The listing builds one solid part. Answer for the finished solid, in the listing's coordinates (mm). Give positions to 0.01 mm unless a question says otherwise; leave off trailing zeros. Order: outer loops, then holes, each group sorted by start corner. A loop starts at its lowest first (then second) coordinate and runs counter-clockwise, first axis right, second up. Notation, with made-up numbers: (44.5, 53) - (53.5, 53) arc R23 ccw to (53.5, 70) - close; hole circle Ø5 at (30, 58.5). An arc over 180 degrees is marked (long way). Answer as CSV lines item,"result". Start each with the question number.
1. Section A-A on z = 0 is taken. Give the vertices of the cut face in (x, y) (3 decimals).
2. Determine the mould class of faces 1 (the flat face through (-8.5, -3, -19)), 2 (the cylindrical face through (-7.3, 17.5, -7.3)), 3 (the cylindrical face through (-7.81, -4.58, 20.65)) for opening direction Y: +Y half, -Y half, draft (parallel to the pull), parting line (faces both ways), or undercut.
3. Flat-ended cylindrical pins translate along their axes: pin 1 (23 mm diameter, centred on y = 0, z = 0, fed in from -X); pin 2 (12 mm diameter, centred on y = 5, z = -11, fed in from +X); pin 3 (6 mm diameter, centred on y = -6.5, z = 13, fed in from +X). Find the tip coordinate at first contact, or state that the pin passes through.
4. Consider line 1 along Z through (x, y) = (-7.2, 0); line 2 along Z through (x, y) = (-8.25, 0). Determine where each line is inside the solid, lowest interval first. Write a range as [from, to].
Solid Edge part; units mm, degrees
sketch "Sketch1" plane through (0, 0, 0) normal (0, 0, 1) x (1, 0, 0)
  line L0 (-8.5, 17.865) -> (-8.5, 17.5)
  line L1 (-8.5, 17.5) -> (-8.1889, 17.5)
  line L2 (-8.1889, 17.5) -> (-7.5667, 18.96)
  line L3 (-7.5667, 18.96) -> (-7.1, 18.96)
  line L4 (-7.1, 18.96) -> (-7.1, 21.15)
  line L5 (-7.1, 21.15) -> (-8.5, 21.15)
  line L6 (-8.5, 21.15) -> (-8.5, 18.96)
  line L7 (-8.5, 18.96) -> (-8.0333, 18.96)
  line L8 (-8.0333, 18.96) -> (-8.5, 17.865)
revolve "RevolvedProtrusion1" add sketch "Sketch1" angle 360 about axis through (17, 0, 0) along (-1, 0, 0)
properties part number "NA 4906UU Seal" material "Aluminio, 7075-T6"
Checks:
1,outline,"(-8.5, -21.15) - (-7.1, -21.15) - (-7.1, -18.96) - (-7.567, -18.96) - (-8.189, -17.5) - (-8.5, -17.5) - (-8.5, -17.865) - (-8.033, -18.96) - (-8.5, -18.96) - close; (-8.5, 17.5) - (-8.189, 17.5) - (-7.567, 18.96) - (-7.1, 18.96) - (-7.1, 21.15) - (-8.5, 21.15) - (-8.5, 18.96) - (-8.033, 18.96) - (-8.5, 17.865) - close"
2,face 1,"draft"
2,face 2,"undercut"
2,face 3,"parting line"
3,pin 1,"passes through"
3,pin 2,"stops at x = -7.94"
3,pin 3,"stops at x = -8.17"
4,line 1,"z = [-21.15, -18.96], [18.96, 21.15]"
4,line 2,"z = [-21.15, -18.96], [-18.45, -17.5], [17.5, 18.45], [18.96, 21.15]"
